from build123d import *

# Parameters (mm, degrees)
INNER_R             = 76.2
BOSS_EXTRUDE1_DEPTH = 13.49375
RIM_R               = 79.375
BOSS_EXTRUDE2_DEPTH = 1.5875
HOLE_R              = 3.175
CUT_EXTRUDE1_DEPTH  = 31.1625


with BuildPart() as part:
    # Inner → Boss-Extrude1 (new body)
    with BuildSketch(Plane.XY):
        Circle(INNER_R)
    extrude(amount=BOSS_EXTRUDE1_DEPTH)

    # Rim → Boss-Extrude2 (add)
    with BuildSketch(Plane.XY.offset(13.49375)):
        Circle(RIM_R)
    extrude(amount=BOSS_EXTRUDE2_DEPTH)

    # Mirror1: part across plane


with BuildPart() as part_1:
    add(part.part)
    add(part.part.mirror(Plane.XY))

    # Hole → Cut-Extrude1 (cut, through all)
    with BuildSketch(Plane.XY.offset(15.08125)):
        Circle(HOLE_R)
    extrude(amount=-CUT_EXTRUDE1_DEPTH, mode=Mode.SUBTRACT)


solid = part_1.part
For this review, take the finished solid that the model builds, in its own axes (mm). A direction names the side the tool comes from. Round coordinates to 2 decimals unless told otherwise and drop trailing zeros. Order: outer loops, then holes, each group sorted by start corner. A loop starts at its lowest first (then second) coordinate and runs counter-clockwise, first axis right, second up. Notation, with made-up numbers: (19.25, 18.25) -> (70.25, 18.25) arc R13 cw to (70.25, 31.25) -> close; hole circle Ø6 at (18, -29.5). An arc over 180 degrees is marked (long way). Put each result on its own line as item: value.
Q1. Mouldability with a two-part tool opening along Z and no side actions: class faces 3 (the flat face through (-71, 30, -13.494)), 4 (the cylindrical face through (75.71, 23.84, -14.28)), 5 (the flat face through (17, 1, 15.081)) as pulls with the +Z half, pulls with the -Z half, needs draft (parallel to the pull), parting line crosses it, or undercut.
Check result:
face 3: undercut
face 4: needs draft
face 5: pulls with the +Z half
Q2. Add section A-A on x = 0. Write out the cut boundary in (y, z) (3 decimals), plus the area to 3 significant figures.
Check result:
outline: (-79.375, -15.081) -> (-3.175, -15.081) -> (-3.175, 15.081) -> (-79.375, 15.081) -> (-79.375, 13.494) -> (-76.2, 13.494) -> (-76.2, -13.494) -> (-79.375, -13.494) -> close; (3.175, -15.081) -> (79.375, -15.081) -> (79.375, -13.494) -> (76.2, -13.494) -> (76.2, 13.494) -> (79.375, 13.494) -> (79.375, 15.081) -> (3.175, 15.081) -> close
area: 4,430 mm2
Q3. Add section D-D on y = -43. Write out the cut boundary in (x, z).
Check result:
outline: (-66.72, -15.08) -> (66.72, -15.08) -> (66.72, -13.49) -> (62.91, -13.49) -> (62.91, 13.49) -> (66.72, 13.49) -> (66.72, 15.08) -> (-66.72, 15.08) -> (-66.72, 13.49) -> (-62.91, 13.49) -> (-62.91, -13.49) -> (-66.72, -13.49) -> close
Q4. Machinability: for faces 1 (the flat face through (17, 1, -15.081)), 2 (the flat face through (-71, 30, 13.494)), which of the approach directions +Z, -Z, +X, -X, +Y, -Y give a long, thin tool a straight path to every point of the face, cutting with its end or side? Answer none if there is none.
Check result:
face 1: -Z, +X, -X, +Y, -Y
face 2: none
Q5. For probe 1 along Y at (x, z) = (0, 9.5) (3 decimals); probe 2 along X at (y, z) = (-38.5, 1); probe 3 along X at (y, z) = (23, -1), list the stretches that pass through material, from the lowest coordinate up. Write a range as [from, to].
Check result:
probe 1: [-76.2, -3.175], [3.175, 76.2]
probe 2: [-65.76, 65.76]
probe 3: [-72.65, 72.65]
Q6. Insertion check: pin 1 Ø1 at (x, z) = (-38.5, -9) entering from -Y; pin 2 Ø2 at (x, z) = (11, -10) entering from +Y; pin 3 Ø1 at (y, z) = (55, 11.5) entering from -X. Each pin has a flat end and moves straight along its axis. Give the tip position at first contact, or say it passes through.
Check result:
pin 1: y = -66.05
pin 2: y = 75.54
pin 3: x = -53.26
Q7. Add section C-C on z = 0.5. Write out the cut boundary in (x, y) (3 decimals), plus the area to 3 significant figures.
Check result:
outline: circle Ø152.4 at (0, 0); hole circle Ø6.35 at (0, 0)
area: 18,200 mm2
